Geometry: see drawing. Coordinates: mm, zero at the bounding-box minimum. A direction names the side the tool comes from. Coordinates: 2 decimals unless noted, no trailing zeros. Order: outer loops, then holes, each group sorted by start corner. A loop starts at its lowest first (then second) coordinate and runs counter-clockwise, first axis right, second up.
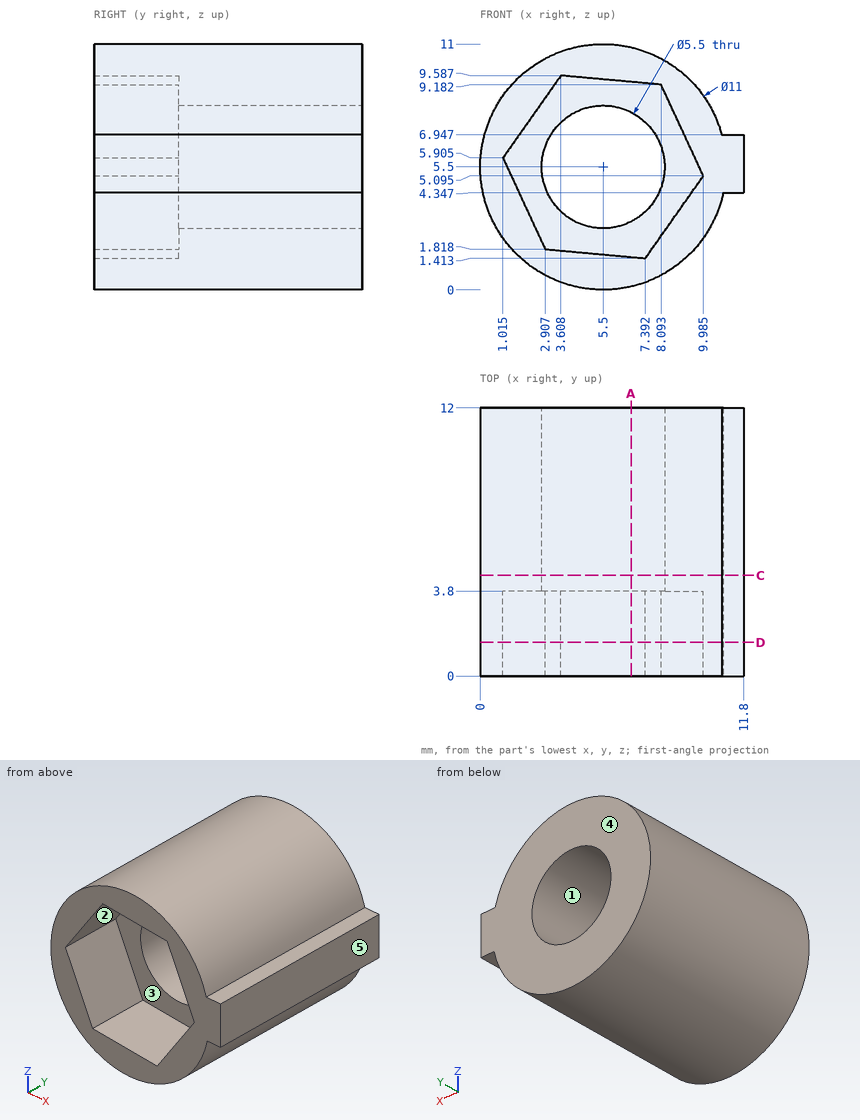
Item 1: Cut plane A-A on x = 6.75. Return loops of the section in (y, z).
Response values:
outline: (0, 0.14) - (12, 0.14) - (12, 3.05) - (3.8, 3.05) - (3.8, 1.47) - (0, 1.47) - close; (0, 9.3) - (3.8, 9.3) - (3.8, 7.95) - (12, 7.95) - (12, 10.86) - (0, 10.86) - close
Item 2: Pin query (flat end, axial travel): pin 1 Ø4 at (y, z) = (8.5, 1.5) entering from +X; pin 2 Ø5 at (x, z) = (5, 8.5) entering from -Y; pin 3 Ø1 at (x, y) = (11, 4.5) entering from -Z; pin 4 Ø3 at (y, z) = (4, 9.5) entering from -X. Return the tip coordinate at first contact, or that it passes through.
Response values:
pin 1: stops at x = 10.62
pin 2: stops at y = 0
pin 3: stops at z = 3.21
pin 4: stops at x = 0.6
Item 3: Cut plane C-C on y = 4.5. Return loops of the section in (x, z).
Response values:
outline: (10.81, 6.95) arc R5.5 ccw (long way) to (10.88, 4.35) - (11.8, 4.35) - (11.8, 6.95) - close; hole circle Ø5.5 at (5.5, 5.5)
Item 4: Ray query, probe 1 along X at (y, z) = (10.25, 5.5); probe 2 along Z at (x, y) = (5.5, 9.75); probe 3 along Y at (x, z) = (3.5, 2.25). Return the intervals inside material, ascending.
Response values:
probe 1: x = 0 to 2.75, 8.25 to 11.8
probe 2: z = 0 to 2.75, 8.25 to 11
probe 3: y = 3.8 to 12
Item 5: Access query for the marked faces 1 and 2. Directions: +Z, -Z, +X, -X, +Y, -Y. A direction counts if a zero-diameter tool reaches every point of the face in a straight line with its end or side. Return the directions, or none.
Response values:
face 1: +Y, -Y
face 2: -Y
Item 6: Cut plane D-D on y = 1.5. Return loops of the section in (x, z) (1 decimal).
Response values:
outline: (10.8, 6.9) arc R5.5 ccw (long way) to (10.9, 4.3) - (11.8, 4.3) - (11.8, 6.9) - close; hole (1, 5.9) - (2.9, 1.8) - (7.4, 1.4) - (10, 5.1) - (8.1, 9.2) - (3.6, 9.6) - close
Item 7: Draft query along X for the marked faces 3, 4 and 5. Return one class per face: pulls with the +X half, pulls with the -X half, needs draft (parallel to the pull), parting line crosses it, or undercut.
Response values:
face 3: undercut
face 4: needs draft
face 5: pulls with the +X half
